```python
from build123d import *

# Parameters (mm, degrees)
MODEL_W                    = 143.05
MODEL_H                    = 122.397505408
MODEL_W_2                  = 14
MODEL_H_2                  = 14
SALIENTE_EXTRUIR1_DEPTH    = 0.75
CROQUIS2_W                 = 15
CROQUIS2_H                 = 30
CORTAR_EXTRUIR1_DEPTH      = 183.633846224
CROQUIS5_W                 = 19.05
CROQUIS5_H                 = 25.819944505
CROQUIS5_W_2               = 17
CROQUIS5_H_2               = 17
SALIENTE_EXTRUIR2_DEPTH    = 2.5
S_LIDO_MOVER_COPIAR1_ANGLE = 180


with BuildPart() as part:
    # Model → Saliente-Extruir1 (new, symmetric)
    with BuildSketch(Plane.XY):
        with Locations((67.525, 57.198752704)):
            Rectangle(MODEL_W, MODEL_H)
        with Locations((58, 42)):
            Rectangle(MODEL_W_2, MODEL_H_2, mode=Mode.SUBTRACT)
        Polygon((18.593146641, 87.427779239), (29.317768845, 78.428752704), (38.316795381, 89.153374907), (27.592173177, 98.152401443), align=None, mode=Mode.SUBTRACT)
        Polygon((103.814404332, 23.723648739), (114.539026536, 14.724622204), (105.54, 4), (94.815377796, 12.999026536), align=None, mode=Mode.SUBTRACT)
        Polygon((33.186293283, 75.182675275), (43.910915486, 66.183648739), (52.909942022, 76.908270943), (42.185319818, 85.907297479), align=None, mode=Mode.SUBTRACT)
        Polygon((20.510973464, 14.724622204), (29.51, 4), (40.234622204, 12.999026536), (31.235595668, 23.723648739), align=None, mode=Mode.SUBTRACT)
        with Locations((77.05, 42)):
            Rectangle(MODEL_W_2, MODEL_H_2, mode=Mode.SUBTRACT)
        Polygon((92.864680182, 85.907297479), (101.863706717, 75.182675275), (91.139084514, 66.183648739), (82.140057978, 76.908270943), align=None, mode=Mode.SUBTRACT)
        Polygon((107.457826823, 98.152401443), (116.456853359, 87.427779239), (105.732231155, 78.428752704), (96.733204619, 89.153374907), align=None, mode=Mode.SUBTRACT)
        Polygon((4, 99.672883204), (14.724622204, 90.673856668), (23.723648739, 101.398478872), (12.999026536, 110.397505408), align=None, mode=Mode.SUBTRACT)
        Polygon((120.325377796, 90.673856668), (111.326351261, 101.398478872), (122.050973464, 110.397505408), (131.05, 99.672883204), align=None, mode=Mode.SUBTRACT)
    extrude(amount=SALIENTE_EXTRUIR1_DEPTH, both=True)

    # Croquis2 → Cortar-Extruir1 (cut, through all)
    with BuildSketch(Plane.XY.offset(0.75)):
        with Locations((67.525, 118.397505408)):
            Rectangle(CROQUIS2_W, CROQUIS2_H)
    extrude(amount=-CORTAR_EXTRUIR1_DEPTH, mode=Mode.SUBTRACT)

    # Croquis5 → Saliente-Extruir2 (add)
    with BuildSketch(Plane(origin=(0, 0, -0.75), x_dir=(-1, 0, 0), z_dir=(0, 0, -1))):
        Polygon((-122.470046698, 115.187534387), (-135.84002898, 99.25380997), (-98.686873488, 68.0786109), (-98.686873488, 23.135715021), (-103.376842573, 28.725002527), (-119.540380323, 15.162183962), (-105.977561759, -1.001353787), (-100.279300069, 3.780055495), (-34.770699931, 3.780055495), (-29.072438241, -1.001353787), (-15.509619677, 15.162183962), (-31.673157427, 28.725002527), (-36.363126512, 23.135715021), (-36.363126512, 68.0786109), (0.79002898, 99.25380997), (-12.579953302, 115.187534387), (-57.699971002, 77.327344177), (-77.350028998, 77.327344177), align=None)
        Polygon((-45.235975991, 12.561464777), (-37.154207116, 5.780055495), (-56, 5.780055495), (-56, 31.6), (-47.6, 31.6), (-47.6, 41), (-38.363126512, 41), (-38.363126512, 20.752207835), align=None, mode=Mode.SUBTRACT)
        with Locations((-67.525, 18.690027748)):
            Rectangle(CROQUIS5_W, CROQUIS5_H, mode=Mode.SUBTRACT)
        Polygon((-79.05, 5.780055495), (-97.895792884, 5.780055495), (-89.814024009, 12.561464777), (-96.686873488, 20.752207835), (-96.686873488, 41), (-87.45, 41), (-87.45, 31.6), (-79.05, 31.6), align=None, mode=Mode.SUBTRACT)
        Polygon((-116.652274615, 14.909507454), (-103.629519082, 25.836896818), (-92.702129717, 12.814141285), (-105.72488525, 1.886751921), align=None, mode=Mode.SUBTRACT)
        with Locations((-77.05, 42)):
            Rectangle(CROQUIS5_W_2, CROQUIS5_H_2, mode=Mode.SUBTRACT)
        Polygon((-42.347870283, 12.814141285), (-31.420480918, 25.836896818), (-18.397725385, 14.909507454), (-29.32511475, 1.886751921), align=None, mode=Mode.SUBTRACT)
        with Locations((-58, 42)):
            Rectangle(CROQUIS5_W_2, CROQUIS5_H_2, mode=Mode.SUBTRACT)
        Polygon((-103.976954796, 74.997790025), (-93.049565432, 88.020545558), (-80.026809899, 77.093156193), (-90.954199263, 64.07040066), align=None, mode=Mode.SUBTRACT)
        Polygon((-133.163248079, 99.487997954), (-122.235858715, 112.510753487), (-109.213103182, 101.583364122), (-120.140492546, 88.560608589), align=None, mode=Mode.SUBTRACT)
        Polygon((-118.570101438, 87.242893989), (-107.642712073, 100.265649522), (-94.61995654, 89.338260158), (-105.547345905, 76.315504625), align=None, mode=Mode.SUBTRACT)
        Polygon((-96.686873488, 66.400411638), (-90.72001128, 61.39361976), (-79.028228261, 75.327344177), (-56.021771739, 75.327344177), (-44.32998872, 61.39361976), (-38.363126512, 66.400411638), (-38.363126512, 43), (-47.6, 43), (-47.6, 52.4), (-87.45, 52.4), (-87.45, 43), (-96.686873488, 43), align=None, mode=Mode.SUBTRACT)
        Polygon((-44.095800737, 64.07040066), (-55.023190101, 77.093156193), (-42.000434568, 88.020545558), (-31.073045204, 74.997790025), align=None, mode=Mode.SUBTRACT)
        Polygon((-29.502654095, 76.315504625), (-40.43004346, 89.338260158), (-27.407287927, 100.265649522), (-16.479898562, 87.242893989), align=None, mode=Mode.SUBTRACT)
        Polygon((-14.909507454, 88.560608589), (-25.836896818, 101.583364122), (-12.814141285, 112.510753487), (-1.886751921, 99.487997954), align=None, mode=Mode.SUBTRACT)
    extrude(amount=SALIENTE_EXTRUIR2_DEPTH)


with BuildPart() as part_1:
    # Sólido-Mover/Copiar1: moved
    add(part.part.rotate(Axis((0, 57.198752704, -0.75), (1, 0, 0)), S_LIDO_MOVER_COPIAR1_ANGLE))


solid = part_1.part
```
Geometry: final body of the model. Coordinates: model frame, mm. A direction names the side the tool comes from. Round coordinates to 2 decimals unless told otherwise and drop trailing zeros. Order: outer loops, then holes, each group sorted by start corner. A loop starts at its lowest first (then second) coordinate and runs counter-clockwise, first axis right, second up. Notation, with made-up numbers: (65.5, 83.5) -> (72.5, 83.5) arc R17 ccw to (72.5, 98.5) -> close; hole circle Ø1 at (7.25, 49). An arc over 180 degrees is marked (long way). Use one line per item in the form item = value. Start each with the question number.
1. Pin query (flat end, axial travel): pin 1 Ø0.8 at (x, z) = (83, 0) entering from +Y; pin 2 Ø0.8 at (y, z) = (58, 0.5) entering from +X; pin 3 Ø2 at (y, z) = (63, 0.5) entering from -X. Return the tip coordinate at first contact, or that it passes through.
2. Reachability of faces 1 (the face through (101.296, 30.682, -1.51)), 2 (the face through (31.961, 112.975, 0.482)), 3 (the face through (34.89, 31.66, 0.48)) from +Z, -Z, +X, -X, +Y, -Y: full face, straight path, thin tool, end or side. Return the list, or none.
3. Line query: probe 1 along Y at (x, z) = (60, 0.6); probe 2 along X at (y, z) = (70.5, 1.4); probe 3 along X at (y, z) = (56, 1.15). Output: solid intervals per line, ascending.
4. Cut plane A-A (y = 44). Return the cut outline in (x, z), then the cut area to 3 significant figures.
5. Cut plane B-B (y = 9). Count the separate pieces of the cut face and the enclosed holes in it, then the cut area to 3 significant figures.
Solution:
q1.pin_1 = 110.62
q1.pin_2 = 98.69
q1.pin_3 = 36.36
q2.face_1 = +Z, -Z
q2.face_2 = +Z, +Y
q2.face_3 = +Z
q3.probe_1 = 37.07 to 39.07, 62 to 63.9, 80.9 to 82.8, 108.62 to 110.62
q3.probe_2 = 36.36 to 38.36, 47.6 to 49.5, 66.5 to 68.55, 85.55 to 87.45, 96.69 to 98.69
q3.probe_3 = 36.36 to 38.36, 96.69 to 98.69
q4.outline = (-4, -2.25) -> (38.89, -2.25) -> (38.89, -0.75) -> (36.56, -0.75) -> (36.56, 1.75) -> (33.6, 1.75) -> (33.6, -0.75) -> (-4, -0.75) -> close; (47.45, -2.25) -> (87.6, -2.25) -> (87.6, -0.75) -> (85.65, -0.75) -> (85.65, 1.75) -> (83.16, 1.75) -> (83.16, -0.75) -> (51.89, -0.75) -> (51.89, 1.75) -> (49.4, 1.75) -> (49.4, -0.75) -> (47.45, -0.75) -> close; (96.16, -2.25) -> (139.05, -2.25) -> (139.05, -0.75) -> (101.45, -0.75) -> (101.45, 1.75) -> (98.49, 1.75) -> (98.49, -0.75) -> (96.16, -0.75) -> close
q4.area = 216 mm^2
q5.separate_pieces = 4
q5.enclosed_holes = 0
q5.area = 189 mm^2
